Model file for the job. Use its own axes, mm. Face numbers are marked on the shaded views. A direction names the side the tool comes from. Round coordinates to 2 decimals unless told otherwise and drop trailing zeros. Order: outer loops, then holes, each group sorted by start corner. A loop starts at its lowest first (then second) coordinate and runs counter-clockwise, first axis right, second up. Notation, with made-up numbers: (71, 31) -> (129, 31) arc R8 cw to (129, 42) -> close; hole circle Ø3 at (28.25, 58). An arc over 180 degrees is marked (long way). Use CSV: the item, a comma, the result in double quotes.
```python
from build123d import *

# Parameters (mm, degrees)
CUT_EXTRUDE1_START = -5
SKETCH2_R          = 22.5
SKETCH2_R_2        = 10
CUT_EXTRUDE1_DEPTH = 5
FILLET1_R          = 1


with BuildPart() as part:
    # Sketch1 → Revolve1 (revolve)
    with BuildSketch(Plane.XY):
        Polygon((0, 5), (0, 30), (2.5, 30), (2.5, 25), (17.5, 25), (17.5, 30), (20, 30), (20, 10), (45, 10), (45, 0), (5, 0), (5, 5), align=None)
    revolve(axis=Axis((45, 0, 0), (-1, 0, 0)))

    # Sketch2 → Cut-Extrude1 (cut)
    with BuildSketch(Plane.ZY.offset(CUT_EXTRUDE1_START)):
        with Locations(Location((0, 0, 0), (0, 0, 270))):
            Circle(SKETCH2_R)
        with Locations(Location((0, 0, 0), (0, 0, 90))):
            Circle(SKETCH2_R_2, mode=Mode.SUBTRACT)
    extrude(amount=CUT_EXTRUDE1_DEPTH, mode=Mode.SUBTRACT)

    # Fillet1
    fillet1_edges = [part.edges().sort_by_distance(p)[0] for p in [
        (0, -10, 0),
    ]]
    fillet(fillet1_edges, radius=FILLET1_R)


solid = part.part
```
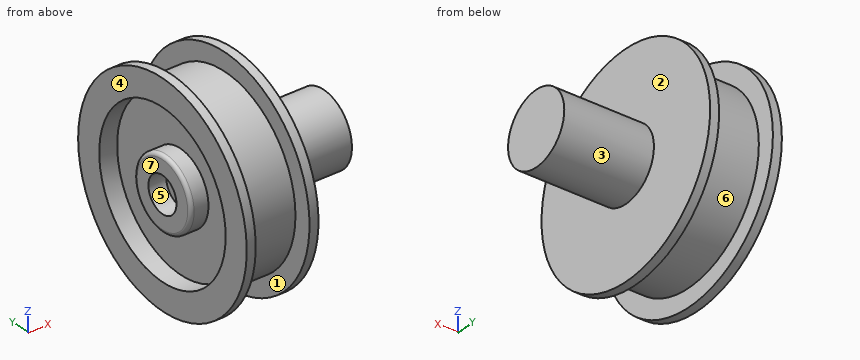
Q1. Cut at D-D (x = 9.5). Give the cut face in (y, z), plus the area to 3 significant figures.
From the geometry:
outline,"circle Ø50 at (0, 0)"
area,"1,960 mm²"
Q2. Probe line 1 along Z through (x, y) = (3.75, 0); line 2 along Z through (x, y) = (1, 0); line 3 along X through (y, z) = (12.5, 25.5). List the from-to ranges inside material, lowest first.
From the geometry:
line 1,"z = -25 to -22.5, -10 to -5, 5 to 10, 22.5 to 25"
line 2,"z = -30 to -22.5, -10 to -5, 5 to 10, 22.5 to 30"
line 3,"x = 0 to 2.5, 17.5 to 20"
Q3. Mould opens along X. For the marked faces 1, 2, 3 and 4 say: +X half, -X half, draft (parallel to the pull), parting line (faces both ways), or undercut.
From the geometry:
face 1,"undercut"
face 2,"+X half"
face 3,"draft"
face 4,"-X half"
Q4. Which spindle directions (+Z, -Z, +X, -X, +Y, -Y) get a long thin tool onto all of the face, cutting with end or side? Do the marked faces 5, 6 and 7. Say none if no direction does.
From the geometry:
face 5,"-X"
face 6,"none"
face 7,"+Z, -Z, -X, +Y, -Y"
Q5. Cut at C-C (x = 35.5). Give the cut face in (y, z), plus the area to 3 significant figures.
From the geometry:
outline,"circle Ø20 at (0, 0)"
area,"314 mm²"
Q6. Pin check, flat tips, straight feed: pin 1 (12 mm diameter, centred on y = -16.5, z = -0.5, fed in from +X); pin 2 (3 mm diameter, centred on y = -1.5, z = 1, fed in from -X); pin 3 (1 mm diameter, centred on x = 16.5, y = 10, fed in from -Z). Stop position of each tip, or through.
From the geometry:
pin 1,"stops at x = 20"
pin 2,"stops at x = 5"
pin 3,"stops at z = -23.12"
